```python
from build123d import *

# Parameters (mm, degrees)
CUT_EXTRUDE2_DEPTH      = 189.478440412
CUT_EXTRUDE2_DEPTH_BACK = 189.478440412
SKETCH3_R               = 21.59
CUT_EXTRUDE3_DEPTH      = 189.478440412
CUT_EXTRUDE3_DEPTH_BACK = 189.478440412
SKETCH4_R               = 5
FILLET1_R               = 2.54


with BuildPart() as part:
    # Sketch1 → Revolve2 (revolve)
    with BuildSketch(Plane.XY, mode=Mode.PRIVATE) as revolve2_sk:
        with BuildLine():
            Line((-39.37, 127), (39.37, 127))
            ThreePointArc((39.37, 127), (51.942358569, 121.792358569), (57.15, 109.22))
            Line((57.15, 109.22), (57.15, 79.564370514))
            ThreePointArc((57.15, 79.564370514), (54.396842649, 70.060560751), (46.99, 63.5))
            Line((46.99, 63.5), (16.51, 49.891733232))
            Line((16.51, 49.891733232), (16.51, 0))
            Line((16.51, 0), (3.796742982, 0))
            Line((3.796742982, 0), (3.796742982, 49.891733232))
            Line((3.796742982, 49.891733232), (-46.99, 63.5))
            ThreePointArc((-46.99, 63.5), (-54.396842649, 70.060560751), (-57.15, 79.564370514))
            Line((-57.15, 79.564370514), (-57.15, 109.22))
            ThreePointArc((-57.15, 109.22), (-51.942358569, 121.792358569), (-39.37, 127))
        make_face()
    revolve(revolve2_sk.sketch.rotate(Axis((3.796742982, 0, 0), (1, 0, 0)), 90), axis=Axis((3.796742982, 0, 0), (1, 0, 0)))

    # Sketch3 → Cut-Extrude2 (cut, two sides: drawn at the far end of the back side and taken through both)
    with BuildSketch(Plane(origin=(0, 0, 0), x_dir=(0, 0, -1), z_dir=(1, 0, 0)).offset(-CUT_EXTRUDE2_DEPTH_BACK)):
        Circle(SKETCH3_R)
    extrude(amount=CUT_EXTRUDE2_DEPTH + CUT_EXTRUDE2_DEPTH_BACK, mode=Mode.SUBTRACT)

    # Sketch4 → Cut-Extrude3 (cut, two sides: drawn at the far end of the back side and taken through both)
    with BuildSketch(Plane(origin=(0, 0, 0), x_dir=(0, 0, -1), z_dir=(1, 0, 0)).offset(-CUT_EXTRUDE3_DEPTH_BACK)):
        with Locations((31.75, 0)):
            Circle(SKETCH4_R)
        with Locations((-15.875, -27.49630657)):
            Circle(SKETCH4_R)
        with Locations((-15.875, 27.49630657)):
            Circle(SKETCH4_R)
    extrude(amount=CUT_EXTRUDE3_DEPTH + CUT_EXTRUDE3_DEPTH_BACK, mode=Mode.SUBTRACT)

    # Fillet1
    fillet1_edges = [part.edges().sort_by_distance(p)[0] for p in [
        (16.51, 0, -49.891733232),
        (3.796742982, 0, -49.891733232),
    ]]
    fillet(fillet1_edges, radius=FILLET1_R)


solid = part.part
```
For this review, take the finished solid that the model builds, in its own axes (mm). A direction names the side the tool comes from. Give positions to 0.01 mm unless a question says otherwise; leave off trailing zeros. Write each loop counter-clockwise with the first axis right and the second up, starting at its lowest first coordinate (ties: lowest second). Pieces come first, ordered by that corner, then holes. Notation, with made-up numbers: M -11,52 L 35,52 A16 ccw 35,73 Z; hole C 89,46.5 d11. An arc over 180 degrees is marked long. Answer as a JSON object with one key per item and string values. Group by question number.
Item 1: For pin 1 Ø3 at (x, z) = (-12, -38.5) entering from -Y; pin 2 Ø1 at (x, z) = (9.5, 7) entering from +Y; pin 3 Ø6 at (y, z) = (27.5, 15.88) entering from -X; pin 4 Ø1.5 at (y, z) = (-30.5, -61) entering from +X, all flat-tipped, find the tip position at first contact; note any pin that passes through.
Item 2: Consider section C-C on x = 10. Write out the cut boundary in (y, z) (3 decimals), plus the area to 3 significant figures.
Item 3: Consider section A-A on z = 0. Write out the cut boundary in (x, y).
Item 4: Draft analysis for pull direction Y (two halves, no side actions). For faces 4 (the cylindrical face through (0.55, 123.98, -27.53)), 5 (the cylindrical face through (10.064, -24.117, 19.56)), 6 (the flat face through (-57.15, 80, -8)), state which applies: +Y half, -Y half, draft (parallel to the pull), parting line (faces both ways), or undercut.
Item 5: Consider section B-B on y = 0. Count the separate pieces of the cut face and the enclosed holes in it, plus the area to 3 significant figures.
Item 6: Consider section D-D on x = 35.5. Write out the cut boundary in (y, z).
Item 7: Tool access review of faces 1 (the cylindrical face through (10.064, 32.454, 16.526)), 2 (the flat face through (16.51, 10, 21)), 3 (the flat face through (3.797, -1, 22)): name each direction out of +Z, -Z, +X, -X, +Y, -Y from which nothing blocks a thin tool from reaching the whole face with its end or side.
Item 8: For probe 1 along X at (y, z) = (110.5, 0); probe 2 along Z at (x, y) = (-33, -47); probe 3 along Y at (x, z) = (19, 16), list the stretches that pass through material, from the lowest coordinate up. Write a range as [from, to].
Check result:
{
 "1": {"pin 1": "stops at y = -121.49", "pin 2": "stops at y = 126.83", "pin 3": "passes through", "pin 4": "stops at x = 53.63"},
 "2": {"outline": "C 0,0 d254; hole C -27.496,15.875 d10; hole C 0,0 d43.18; hole C 0,-31.75 d10; hole C 27.496,15.875 d10", "area": "49,000 mm^2"},
 "3": {"outline": "M -57.15,-109.22 A17.78 ccw -39.37,-127 L 39.37,-127 A17.78 ccw 57.15,-109.22 L 57.15,-79.56 A17.78 ccw 46.99,-63.5 L 18.01,-50.56 A2.54 cw 16.51,-48.24 L 16.51,-21.59 L 3.8,-21.59 L 3.8,-47.94 A2.54 cw 1.91,-50.4 L -46.99,-63.5 A17.78 ccw -57.15,-79.56 Z; M -57.15,79.56 A17.78 ccw -46.99,63.5 L 1.91,50.4 A2.54 cw 3.8,47.94 L 3.8,21.59 L 16.51,21.59 L 16.51,48.24 A2.54 cw 18.01,50.56 L 46.99,63.5 A17.78 ccw 57.15,79.56 L 57.15,109.22 A17.78 ccw 39.37,127 L -39.37,127 A17.78 ccw -57.15,109.22 Z"},
 "4": {"face 4": "parting line", "face 5": "undercut", "face 6": "draft"},
 "5": {"separate pieces": "3", "enclosed holes": "0", "area": "16,100 mm^2"},
 "6": {"outline": "C 0,0 d254; hole C 0,0 d116.74"},
 "7": {"face 1": "+X, -X", "face 2": "+X", "face 3": "-X"},
 "8": {"probe 1": "x = [-57.1, 57.1]", "probe 2": "z = [-117.98, -36.89], [36.89, 117.98]", "probe 3": "y = [-125.99, -48.43], [48.43, 125.99]"}
}
